Geometry: final body of the model. Coordinates: model frame, mm. A direction names the side the tool comes from. Give positions to 0.01 mm unless a question says otherwise; leave off trailing zeros. Order: outer loops, then holes, each group sorted by start corner. A loop starts at its lowest first (then second) coordinate and runs counter-clockwise, first axis right, second up. Notation, with made-up numbers: (66, -31) -> (121, -31) arc R18 cw to (121, 4) -> close; hole circle Ø9 at (74.5, -19). An arc over 180 degrees is marked (long way). One line per question, with ' | ' between items.
from build123d import *

# Parameters (mm, degrees)
F0_R     = 2.159
F0_W     = 40.3
F0_H     = 20.2184
F1_DEPTH = 3.175


# Not quite as in the source:
# - a length typed as a fraction of an inch, garbled in the dataset ("3 / 203.2 mm" for 3/8 in), is restored


with BuildPart() as f1:
    # F0 (on Top) → F1 (new body)
    with BuildSketch(Plane.XY):
        Polygon((28.575, -19.1008), (28.575, 12.6492), (-28.575, 12.6492), (-28.575, -19.1008), (-15.875, -19.1008), (-15.875, -22.2758), (-9.525, -22.2758), (-9.525, -19.1008), (-1.524, -19.1008), (-1.524, -16.764), (-2.38125, -16.764), (-2.38125, -15.0876), (-1.524, -15.0876), (-1.524, -12.7508), (1.524, -12.7508), (1.524, -15.0876), (2.38125, -15.0876), (2.38125, -16.764), (1.524, -16.764), (1.524, -19.1008), (9.525, -19.1008), (9.525, -22.2758), (15.875, -22.2758), (15.875, -19.1008), align=None)
        with Locations((-23.96, -4.3434)):
            Circle(F0_R, mode=Mode.SUBTRACT)
        with Locations((-23.96, 4.3434)):
            Circle(F0_R, mode=Mode.SUBTRACT)
        Rectangle(F0_W, F0_H, mode=Mode.SUBTRACT)
        with Locations((23.96, -4.3434)):
            Circle(F0_R, mode=Mode.SUBTRACT)
        with Locations((23.96, 4.3434)):
            Circle(F0_R, mode=Mode.SUBTRACT)
    extrude(amount=F1_DEPTH)


solid = f1.part
1) Section B-B on y = -8.5. Return loops of the section in (x, z) (3 decimals), plus the area to 3 significant figures.
Check result:
outline: (-28.575, 0) -> (-20.15, 0) -> (-20.15, 3.175) -> (-28.575, 3.175) -> close; (20.15, 0) -> (28.575, 0) -> (28.575, 3.175) -> (20.15, 3.175) -> close | area: 53.5 mm^2
2) Set-up query: faces 1 (the flat face through (0, -12, 0)), 2 (the flat face through (0, -10.109, 2)), 3 (the flat face through (9.525, -21, 2)). Return all of +Z, -Z, +X, -X, +Y, -Y with unobstructed straight access to the full face (end or side cutting, diameter ignored); none if empty.
Check result:
face 1: -Z, +X, -X, +Y, -Y | face 2: +Z, -Z | face 3: +Z, -Z, -Y
3) Material intervals for probe 1 along Y at (x, z) = (-23.96, 1); probe 2 along X at (y, z) = (-13, 1.9) (3 decimals); probe 3 along X at (y, z) = (-16.5, 1.6) (3 decimals), sorted ascending. Write a range as from..to.
Check result:
probe 1: y = -19.1..-6.5, -2.18..2.18, 6.5..12.65 | probe 2: x = -28.575..-1.524, 1.524..28.575 | probe 3: x = -28.575..-2.381, 2.381..28.575
4) Contact query for flat-ended pins moving along their axis: pin 1 Ø8 at (x, y) = (19, -15.5) entering from -Z; pin 2 Ø1 at (x, z) = (4.5, 2) entering from -Y; pin 3 Ø1.6 at (y, z) = (-21, 1) entering from +X (3 decimals). Output: stop coordinate, or through.
Check result:
pin 1: stops at z = 0 | pin 2: stops at y = -19.1 | pin 3: stops at x = 15.875
5) Section A-A on x = -18. Return loops of the section in (y, z) (3 decimals), plus the area to 3 significant figures.
Check result:
outline: (-19.101, 0) -> (-10.109, 0) -> (-10.109, 3.175) -> (-19.101, 3.175) -> close; (10.109, 0) -> (12.649, 0) -> (12.649, 3.175) -> (10.109, 3.175) -> close | area: 36.6 mm^2
6) Pull-direction query (X, two-part tool) for faces 4 (the flat face through (-22, -19.101, 2)), 5 (the flat face through (-1.524, -14, 2)), 6 (the flat face through (-28.575, -3, 2)); classes: +X half, -X half, draft (parallel to the pull), parting line (faces both ways), or undercut.
Check result:
face 4: draft | face 5: undercut | face 6: -X half
7) Section C-C on x = -23.96. Return loops of the section in (y, z) (3 decimals), plus the area to 3 significant figures.
Check result:
outline: (-19.101, 0) -> (-6.502, 0) -> (-6.502, 3.175) -> (-19.101, 3.175) -> close; (-2.184, 0) -> (2.184, 0) -> (2.184, 3.175) -> (-2.184, 3.175) -> close; (6.502, 0) -> (12.649, 0) -> (12.649, 3.175) -> (6.502, 3.175) -> close | area: 73.4 mm^2
8) Section D-D on z = 1.6. Count the separate pieces of the cut face and the enclosed holes in it, plus the area to 3 significant figures.
Check result:
separate pieces: 1 | enclosed holes: 5 | area: 959 mm^2
